from build123d import *

# Parameters (mm, degrees)
SKETCH1_R           = 8
BOSS_EXTRUDE1_DEPTH = 3.9
SKETCH2_R           = 9
BOSS_EXTRUDE2_DEPTH = 1.1
SKETCH3_R           = 6.75
SKETCH3_R_2         = 5
CUT_EXTRUDE1_DEPTH  = 0.5
SKETCH3_3_R         = 4
CUT_EXTRUDE2_DEPTH  = 14.674794331


with BuildPart() as part:
    # Sketch1 → Boss-Extrude1 (new body)
    with BuildSketch(Plane.XY):
        Circle(SKETCH1_R)
    extrude(amount=BOSS_EXTRUDE1_DEPTH)

    # Sketch2 → Boss-Extrude2 (add)
    with BuildSketch(Plane.XY.offset(3.9)):
        Circle(SKETCH2_R)
    extrude(amount=BOSS_EXTRUDE2_DEPTH)

    # Sketch3 → Cut-Extrude1 (cut)
    with BuildSketch(Plane(origin=(0, 0, 0), x_dir=(-1, 0, 0), z_dir=(0, 0, -1))):
        Circle(SKETCH3_R)
        Circle(SKETCH3_R_2, mode=Mode.SUBTRACT)
    cut_extrude1 = extrude(amount=-CUT_EXTRUDE1_DEPTH, mode=Mode.SUBTRACT)

    # Sketch3<3> → Cut-Extrude2 (cut, through all)
    with BuildSketch(Plane(origin=(0, 0, 0), x_dir=(-1, 0, 0), z_dir=(0, 0, -1))):
        Circle(SKETCH3_3_R)
    extrude(amount=-CUT_EXTRUDE2_DEPTH, mode=Mode.SUBTRACT)

    # Mirror1: Cut-Extrude1 across plane
    add(cut_extrude1.mirror(Plane(origin=(0, 0, 2.5), x_dir=(1, 0, 0), z_dir=(0, 0, -1))), mode=Mode.SUBTRACT)


solid = part.part
Can you work these out from the model? Positions are in its coordinate system, mm. A direction names the side the tool comes from. Round coordinates to 2 decimals unless told otherwise and drop trailing zeros. Order: outer loops, then holes, each group sorted by start corner. A loop starts at its lowest first (then second) coordinate and runs counter-clockwise, first axis right, second up. Notation, with made-up numbers: (66.5, -34.75) -> (113.5, -34.75) arc R16 cw to (113.5, -19.75) -> close; hole circle Ø3 at (-20.5, 71). An arc over 180 degrees is marked (long way). Write each question's results on one line, items separated by ' | '. Start each with the question number.
Item 1: If we section it at C-C, the plane x = 7.75: Write out the boundary of the cut face in (y, z), then the cut area to 3 significant figures.
Item 2: Please list where these lines run through material, in increasing order: L1, parallel to Y at x = 0, z = 4.6; L2, parallel to Y at x = 0, z = 0.45; L3, parallel to X at y = 1, z = 4.8.
Item 3: If we section it at D-D, the plane z = 1: Write out the boundary of the cut face in (x, y), then the cut area to 3 significant figures.
Item 4: Which directions (+Z, -Z, +X, -X, +Y, -Y) give clear straight access to the entire face, cutting with the end or side of a thin tool? Please do faces 1 (the cylindrical face through (1.46, -6.59, 0.25)), 2 (the flat face through (-4, -6, 0)), 3 (the flat face through (5, -2, 4.5)).
Item 5: Thinking about a two-plate mould opening in Y: for faces 4 (the cylindrical face through (1.08, -4.88, 4.75)), 5 (the cylindrical face through (1.08, -4.88, 0.25)), 6 (the flat face through (1, 7, 5)), 7 (the cylindrical face through (-1.73, -7.81, 1.92)), which applies, +Y half, -Y half, draft (parallel to the pull), parting line (faces both ways), or undercut?
Item 6: If we section it at A-A, the plane y = 0: Write out the boundary of the cut face in (x, z).
Item 7: Will this pin go through, and if not, where does the flat tip stop? pin 1 (5 mm diameter, centred on x = 0, y = 0, fed in from -Z).
Results:
1) outline: (-4.58, 3.9) -> (-1.98, 3.9) -> (-1.98, 0) -> (1.98, 0) -> (1.98, 3.9) -> (4.58, 3.9) -> (4.58, 5) -> (-4.58, 5) -> close | area: 25.5 mm2
2) L1: y = -9 to -6.75, -5 to -4, 4 to 5, 6.75 to 9 | L2: y = -8 to -6.75, -5 to -4, 4 to 5, 6.75 to 8 | L3: x = -8.94 to -6.68, -4.9 to -3.87, 3.87 to 4.9, 6.68 to 8.94
3) outline: circle Ø16 at (0, 0); hole circle Ø8 at (0, 0) | area: 151 mm2
4) face 1: -Z | face 2: -Z, +X, -X, +Y, -Y | face 3: +Z
5) face 4: undercut | face 5: undercut | face 6: draft | face 7: parting line
6) outline: (-9, 3.9) -> (-8, 3.9) -> (-8, 0) -> (-6.75, 0) -> (-6.75, 0.5) -> (-5, 0.5) -> (-5, 0) -> (-4, 0) -> (-4, 5) -> (-5, 5) -> (-5, 4.5) -> (-6.75, 4.5) -> (-6.75, 5) -> (-9, 5) -> close; (4, 0) -> (5, 0) -> (5, 0.5) -> (6.75, 0.5) -> (6.75, 0) -> (8, 0) -> (8, 3.9) -> (9, 3.9) -> (9, 5) -> (6.75, 5) -> (6.75, 4.5) -> (5, 4.5) -> (5, 5) -> (4, 5) -> close
7) pin 1: passes through
